Autodesk Inventor part; units mm, degrees
ref_plane "YZ Plane" through (0, 0, 0) normal (1, 0, 0) x (0, 1, 0)
ref_plane "XZ Plane" through (0, 0, 0) normal (0, 1, 0) x (-1, 0, 0)
ref_plane "XY Plane" through (0, 0, 0) normal (0, 0, 1) x (1, 0, 0)
sketch "Sketch1" plane through (0, 0, 0) normal (1, 0, 0) x (0, 1, 0)
  line L0 (0, 25.4) -> (0, 0)
  line L1 (0, 25.4) -> (609.6, 25.4)
  line L2 (609.6, 25.4) -> (681.442, 97.242)
  line L3 (681.442, 97.242) -> (632.8429, 48.6429)
  line L4 (681.442, 97.242) -> (699.4026, 79.2815)
  line L5 (699.4026, 79.2815) -> (620.121, 0)
  line L6 (0, 0) -> (620.121, 0)
  line L7 (609.6, 25.4) -> (620.121, 0) construction
  circle A0 centre (614.8605, 12.7) radius 6.35
  circle A1 centre (681.442, 79.2815) radius 3.175
  dimension "d0" = 25.4
  dimension "d7" = 609.6
  dimension "d8" = 101.6
  dimension "d9" = 135
  dimension "d10" = 25.4
  dimension "d11" = 12.7
  dimension "d12" = 6.35
  dimension "d13" = 12.7
  dimension "d14" = 12.7
extrude "Extrusion1" add sketch "Sketch1" along normal blind 6.35
properties part number "Cart Handle"
The model under review builds one solid part; all positions refer to its coordinate system, in mm. Give positions to 0.01 mm unless a question says otherwise; leave off trailing zeros. Write each loop counter-clockwise with the first axis right and the second up, starting at its lowest first coordinate (ties: lowest second). Pieces come first, ordered by that corner, then holes. Notation, with made-up numbers: M -39.75,39 L -20.75,39 A23 ccw -20.75,67 Z; hole C 46.5,82.5 d10. An arc over 180 degrees is marked long. One line per question, with ' | ' between items. Start each with the question number.
Item 1: For pin 1 (3 mm diameter, centred on x = 3.5, y = 626.5, fed in from +Z); pin 2 (3 mm diameter, centred on x = 3, y = 200.5, fed in from +Z); pin 3 (5 mm diameter, centred on y = 681.44, z = 79.28, fed in from +X) (3 decimals); pin 4 (2 mm diameter, centred on x = 2.5, z = 74, fed in from +Y), all flat-tipped, find the tip position at first contact; note any pin that passes through.
Item 2: We need section B-B on x = 3.25. Give the number of separate pieces and of enclosed holes in the cut face, plus the area to 3 significant figures.
Item 3: We need section C-C on y = 599.5. Write out the cut boundary in (x, z).
Item 4: We need section D-D on z = 63. Write out the cut boundary in (x, y), plus the area to 3 significant figures.
Item 5: We need section A-A on z = 12.7. Write out the cut boundary in (x, y), plus the area to 3 significant figures.
Item 6: Draft analysis for pull direction Z (two halves, no side actions). For faces 1 (the flat face through (3.13, 660.32, 40.2)), 2 (the flat face through (6.35, 348, 16)), 3 (the cylindrical face through (3.13, 609.82, 16.56)), 4 (the flat face through (3.131, 690.297, 88.387)), state which applies: released by +Z, released by -Z, zero draft, split by the parting line, or undercut.
Item 7: Wall thickness on line 1 (Z direction, x = 4.25, y = 571.5); line 2 (Y direction, x = 2, z = 7.5); line 3 (Y direction, x = 5.75, z = 8.5): over which ranges is each line inside the solid? List them lowest first. Write a range as from..to.
Results found:
1) pin 1: stops at z = 43.8 | pin 2: stops at z = 25.4 | pin 3: passes through | pin 4: stops at y = 695.12
2) separate pieces: 1 | enclosed holes: 2 | area: 18,200 mm2
3) outline: M 0,0 L 6.35,0 L 6.35,25.4 L 0,25.4 Z
4) outline: M 0,647.2 L 6.35,647.2 L 6.35,683.12 L 0,683.12 Z | area: 228 mm2
5) outline: M 0,0 L 6.35,0 L 6.35,608.51 L 0,608.51 Z; M 0,621.21 L 6.35,621.21 L 6.35,632.82 L 0,632.82 Z | area: 3,940 mm2
6) face 1: released by -Z | face 2: zero draft | face 3: undercut | face 4: released by +Z
7) line 1: z = 0..25.4 | line 2: y = 0..611.22, 618.51..627.62 | line 3: y = 0..610.1, 619.62..628.62
